Could you check a few things on this model? Use its own coordinates, in mm. Give positions to 0.01 mm unless a question says otherwise; leave off trailing zeros. Write each loop counter-clockwise with the first axis right and the second up, starting at its lowest first coordinate (ties: lowest second). Pieces come first, ordered by that corner, then holes. Notation, with made-up numbers: (39, 3.25) -> (47, 3.25) arc R22 ccw to (47, 25.25) -> close; hole circle Ø6 at (34.5, 21.25). An arc over 180 degrees is marked (long way). One line per question, with ' | ' between items.
from build123d import *

# Parameters (mm, degrees)
SKETCH1_R           = 171
BOSS_EXTRUDE1_DEPTH = 10
SKETCH2_R           = 141
CUT_EXTRUDE1_DEPTH  = 11
BOSS_EXTRUDE2_DEPTH = 15
BOSS_EXTRUDE3_DEPTH = 15


with BuildPart() as part:
    # Sketch1 → Boss-Extrude1 (new body)
    with BuildSketch(Plane(origin=(0, 0, 0), x_dir=(1, 0, 0), z_dir=(0, 1, 0))):
        Circle(SKETCH1_R)
    extrude(amount=BOSS_EXTRUDE1_DEPTH)

    # Sketch2 → Cut-Extrude1 (cut, through all)
    with BuildSketch(Plane(origin=(0, 10, 0), x_dir=(1, 0, 0), z_dir=(0, 1, 0))):
        Circle(SKETCH2_R)
    extrude(amount=-CUT_EXTRUDE1_DEPTH, mode=Mode.SUBTRACT)

    # Sketch3 → Boss-Extrude2 (add)
    with BuildSketch(Plane.XZ):
        with BuildLine():
            Line((29.693838381, 168.402125765), (29.172893848, 165.447702506))
            ThreePointArc((29.172893848, 165.447702506), (14.689274555, 167.356581027), (0.094580612, 167.999973377))
            ThreePointArc((0.094580612, 167.999973377), (-14.547941757, 167.368926001), (-29.079745505, 165.464100038))
            Line((-29.079745505, 165.464100038), (-29.730542301, 168.395649749))
            ThreePointArc((-29.730542301, 168.395649749), (-14.940760682, 170.346040959), (-0.037270853, 170.999995938))
            ThreePointArc((-0.037270853, 170.999995938), (14.885067408, 170.350916547), (29.693838381, 168.402125765))
        make_face()
    extrude(amount=BOSS_EXTRUDE2_DEPTH)

    # Sketch4 → Boss-Extrude3 (add)
    with BuildSketch(Plane.XZ):
        with BuildLine():
            Line((29.712190517, -168.398888757), (29.120639245, -165.456907894))
            ThreePointArc((29.120639245, -165.456907894), (14.566625791, -167.367300907), (-0.098592842, -167.99997107))
            ThreePointArc((-0.098592842, -167.99997107), (-14.740379926, -167.352087527), (-29.269983819, -165.430553548))
            Line((-29.269983819, -165.430553548), (-29.675485892, -168.405360773))
            ThreePointArc((-29.675485892, -168.405360773), (-14.885067408, -170.350916547), (0.018635427, -170.999998985))
            ThreePointArc((0.018635427, -170.999998985), (14.922196434, -170.347668178), (29.712190517, -168.398888757))
        make_face()
    extrude(amount=BOSS_EXTRUDE3_DEPTH)


solid = part.part
Q1. If I drill on line 1 along X through (y, z) = (4.25, 0); line 2 along Y through (x, z) = (13, -141), over which ranges is the centre line in solid material (lowest first)?
Answer below:
line 1: x = -171 to -141, 141 to 171 | line 2: y = 0 to 10
Q2. Imagine slicing it at D-D on z = 149.5. Please give me the cut outline in (x, y), and give its area (3 significant figures).
Answer below:
outline: (-83.01, 0) -> (83.01, 0) -> (83.01, 10) -> (-83.01, 10) -> close | area: 1,660 mm^2
Q3. Imagine slicing it at B-B on z = 0. Please give me the cut outline in (x, y).
Answer below:
outline: (-171, 0) -> (-141, 0) -> (-141, 10) -> (-171, 10) -> close; (141, 0) -> (171, 0) -> (171, 10) -> (141, 10) -> close
Q4. Imagine slicing it at C-C on x = -137. Please give me the cut outline in (y, z), and give its area (3 significant figures).
Answer below:
outline: (0, -102.33) -> (10, -102.33) -> (10, -33.35) -> (0, -33.35) -> close; (0, 33.35) -> (10, 33.35) -> (10, 102.33) -> (0, 102.33) -> close | area: 1,380 mm^2
Q5. Imagine slicing it at A-A on y = -6.5. Please give me the cut outline in (x, z), and give its area (3 significant figures).
Answer below:
outline: (-29.73, 168.4) -> (-29.08, 165.46) arc R168 cw to (29.17, 165.45) -> (29.69, 168.4) arc R171 ccw to start; (-29.68, -168.41) arc R171 ccw to (29.71, -168.4) -> (29.12, -165.46) arc R168 cw to (-29.27, -165.43) -> close | area: 355 mm^2
Q6. If we mould it in two halves opening along Z, with no side actions, what happens to faces 1 (the cylindrical face through (-111.89, 5.07, 85.8)), 2 (the flat face through (25, 10, -140))? For each: +Z half, -Z half, draft (parallel to the pull), parting line (faces both ways), or undercut.
Answer below:
face 1: undercut | face 2: draft
Q7. Will these pins go through, and if not, where does the flat tip stop? pin 1 (5 mm diameter, centred on y = 6.5, z = -68, fed in from +X); pin 2 (1 mm diameter, centred on y = 6.5, z = -55, fed in from +X); pin 3 (4 mm diameter, centred on y = 5.5, z = 105.5, fed in from -X).
Answer below:
pin 1: stops at x = 157.96 | pin 2: stops at x = 162.08 | pin 3: stops at x = -136.12
